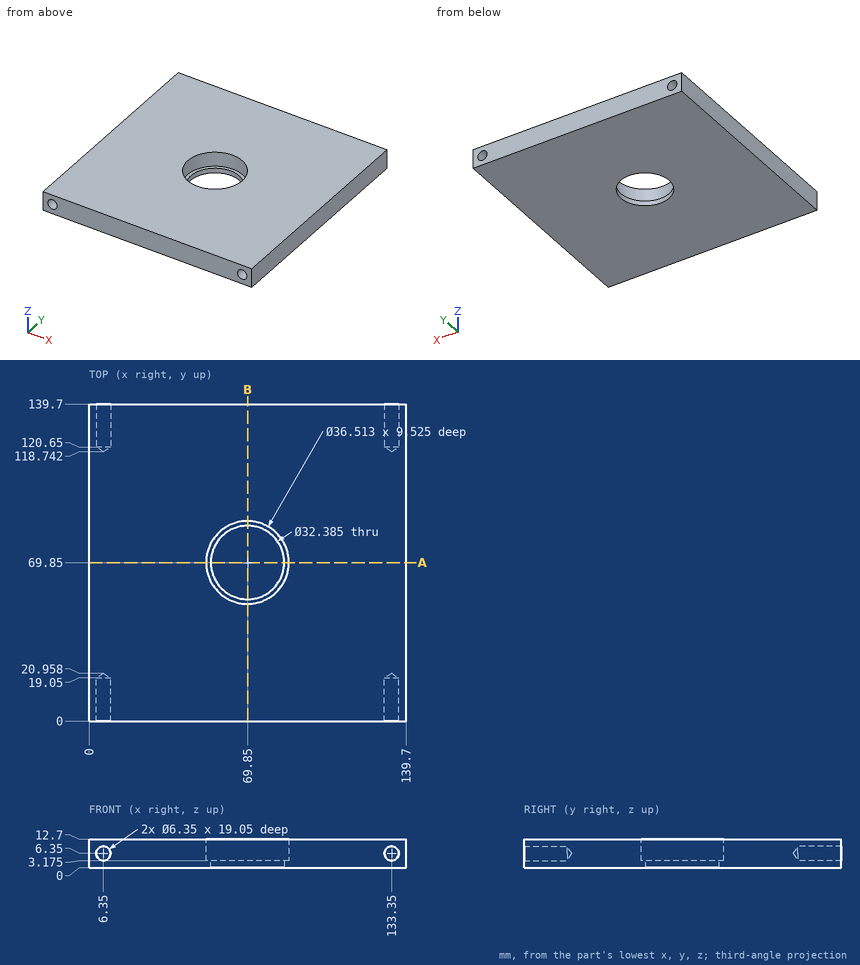
The figure shows three views and two pictorial views of one solid part (mm, origin at its lowest corner). Answer the questions. Give positions to 0.01 mm unless a question says otherwise; leave off trailing zeros. Order: outer loops, then holes, each group sorted by start corner. A loop starts at its lowest first (then second) coordinate and runs counter-clockwise, first axis right, second up. Notation, with made-up numbers: (30.5, 45) -> (65.5, 45) arc R21 ccw to (65.5, 83) -> close; hole circle Ø1 at (60, -16). An arc over 180 degrees is marked (long way). Answer as a JSON object with one key per item and string values. Group by question number.
Item 1: The part is cut by section A-A on y = 69.85. Write down the section's boundary in (x, z) (1 decimal), and give its area (3 significant figures).
Item 2: Consider L1, parallel to X at y = 126, z = 6.35 (1 decimal); L2, parallel to Z at x = 6, y = 129 (1 decimal); L3, parallel to Y at x = 69.85, z = 8.5. Determine where each line is inside the solid, lowest interval first. Write a range as from..to.
Item 3: Flat-ended cylindrical pins translate along their axes: pin 1 (4 mm diameter, centred on x = 133.35, z = 6.35, fed in from -Y) (1 decimal); pin 2 (5.5 mm diameter, centred on x = 6.35, z = 6.35, fed in from -Y) (1 decimal); pin 3 (5 mm diameter, centred on x = 133.35, z = 6.35, fed in from +Y) (1 decimal). Find the tip coordinate at first contact, or state that the pin passes through.
Result set:
{
 "1": {"outline": "(0, 0) -> (53.7, 0) -> (53.7, 3.2) -> (51.6, 3.2) -> (51.6, 12.7) -> (0, 12.7) -> close; (86, 0) -> (139.7, 0) -> (139.7, 12.7) -> (88.1, 12.7) -> (88.1, 3.2) -> (86, 3.2) -> close", "area": "1,320 mm²"},
 "2": {"L1": "0..3.2, 9.5..130.2, 136.5..139.7", "L2": "0..3.2, 9.5..12.7", "L3": "0..51.59, 88.11..139.7"},
 "3": {"pin 1": "y = 19.8", "pin 2": "y = 19.3", "pin 3": "y = 120.2"}
}
